Source: CAD feature listing. Evaluate the final solid. Frame: model axes, mm. Give positions to 0.01 mm unless a question says otherwise; leave off trailing zeros. Write each loop counter-clockwise with the first axis right and the second up, starting at its lowest first coordinate (ties: lowest second). Pieces come first, ordered by that corner, then holes.
Autodesk Inventor part; units mm, degrees
ref_plane "YZ Plane" through (0, 0, 0) normal (1, 0, 0) x (0, 1, 0)
ref_plane "XZ Plane" through (0, 0, 0) normal (0, 1, 0) x (-1, 0, 0)
ref_plane "XY Plane" through (0, 0, 0) normal (0, 0, 1) x (1, 0, 0)
sketch "Sketch1" plane through (0, 0, 0) normal (0, 1, 0) x (-1, 0, 0)
  line L0 (25.4, 25.4) -> (-25.4, 25.4)
  line L1 (-25.4, 25.4) -> (-25.4, -25.4)
  line L2 (-25.4, -25.4) -> (25.4, -25.4)
  line L3 (25.4, -25.4) -> (25.4, 25.4)
  point P0 (0, 0)
  dimension "d0" = 50.8
  dimension "d1" = 50.8
  dimension "d2" = 25.4
  dimension "d3" = 25.4
extrude "Extrusion1" add sketch "Sketch1" along normal blind 6.35
sketch "Sketch2" plane through (0, 6.35, 0) normal (0, 1, 0) x (1, 0, 0)
  point P0 (0, 0)
  point P1 (-19.05, -19.05)
  point P2 (-19.05, 19.05)
  point P3 (19.05, 19.05)
  point P4 (19.05, -19.05)
  dimension "d6" = 38.1
  dimension "d7" = 38.1
  dimension "d8" = 19.05
  dimension "d9" = 19.05
hole "Hole1" at (-19.05, 6.35, 19.05) at (-19.05, 6.35, -19.05) at (19.05, 6.35, -19.05) at (19.05, 6.35, 19.05) direction (0, -1, 0) diameter 6.7564 end through all
fillet "Fillet1" radius 3.175 4 edges at (-25.4, 3.175, 25.4) (-25.4, 3.175, -25.4) (25.4, 3.175, -25.4) (25.4, 3.175, 25.4)
sketch "Sketch3" plane through (0, 6.35, 0) normal (0, 1, 0) x (1, 0, 0)
  point P0 (0, 0)
  point P1 (0, 0)
hole "Hole2" at (0, 6.35, 0) direction (0, -1, 0) diameter 13.4874 end through all
properties part number "Motor_Shaft_Attachment"
1. Line query: L1, parallel to X at y = 3.5, z = -19.05; L2, parallel to X at y = 4.5, z = 21. Output: solid intervals per line, ascending.
2. Cut plane D-D, the plane z = -19.05. Return the cut outline in (x, y).
3. Contact query for a flat-ended pin moving along its axis: P1, Ø11, axis at x = -19.05, z = -19.05, coming from the +Y side. Output: stop coordinate, or through.
4. Mould query, pull axis Z, two halves, no side actions, for faces 1 (the cylindrical face through (24.49, 3.22, -24.45)), 2 (the cylindrical face through (16.201, 3.131, 20.866)), 3 (the cylindrical face through (24.45, 3.22, 24.49)). Classes: +Z half, -Z half, draft (parallel to the pull), parting line (faces both ways), or undercut.
5. Cut plane C-C, the plane x = 19.05. Return the cut outline in (y, z).
6. Cut plane A-A, the plane z = 0. Return the cut outline in (x, y), then the cut area to 3 significant figures.
7. Cut plane B-B, the plane x = 0. Return the cut outline in (y, z).
Response values:
1. L1: x = -25.4 to -22.43, -15.67 to 15.67, 22.43 to 25.4
1. L2: x = -25.4 to -21.81, -16.29 to 16.29, 21.81 to 25.4
2. outline: (-25.4, 0) - (-22.43, 0) - (-22.43, 6.35) - (-25.4, 6.35) - close; (-15.67, 0) - (15.67, 0) - (15.67, 6.35) - (-15.67, 6.35) - close; (22.43, 0) - (25.4, 0) - (25.4, 6.35) - (22.43, 6.35) - close
3. P1: stops at y = 6.35
4. face 1: -Z half
4. face 2: undercut
4. face 3: +Z half
5. outline: (0, -25.4) - (6.35, -25.4) - (6.35, -22.43) - (0, -22.43) - close; (0, -15.67) - (6.35, -15.67) - (6.35, 15.67) - (0, 15.67) - close; (0, 22.43) - (6.35, 22.43) - (6.35, 25.4) - (0, 25.4) - close
6. outline: (-25.4, 0) - (-6.74, 0) - (-6.74, 6.35) - (-25.4, 6.35) - close; (6.74, 0) - (25.4, 0) - (25.4, 6.35) - (6.74, 6.35) - close
6. area: 237 mm2
7. outline: (0, -25.4) - (6.35, -25.4) - (6.35, -6.74) - (0, -6.74) - close; (0, 6.74) - (6.35, 6.74) - (6.35, 25.4) - (0, 25.4) - close
